Design review of the part built by this model. Coordinates are the model's own, in mm. Coordinates: 2 decimals unless noted, no trailing zeros. Loops run counter-clockwise (first coordinate to the right, second up) from the corner with the lowest first, then second, coordinate; pieces in that order, holes last. Notation, with made-up numbers: (1, 21.25) -> (20, 21.25) arc R10 cw to (20, 26.25) -> close; hole circle Ø6 at (5, 84). An arc over 180 degrees is marked (long way). Use a Markdown table: item, result. Add a question column.
Q1. For probe 1 along Y at (x, z) = (-50, 3.75); probe 2 along X at (y, z) = (38.5, 0.6); probe 3 along Y at (x, z) = (31, 1.25), list the stretches that pass through material, from the lowest coordinate up.
Q2. Take a section at B-B on y = -53. Write out the cut boundary in (x, z), plus the area to 3 significant figures.
Q3. Take a section at A-A on x = 7.5. Write out the cut boundary in (y, z).
Q4. Take a section at D-D on y = -20. Write out the cut boundary in (x, z).
Q5. Take a section at C-C on z = 4.55. Count the separate pieces of the cut face and the enclosed holes in it, plus the area to 3 significant figures.
Q6. Clearance check with a flat-ended pin moving along its axis: pin 1 Ø4.5 at (x, y) = (30, 40) entering from +Z. State where the tip first meets the part, or that it passes through.
Q7. Draft analysis for pull direction X (two halves, no side actions). For faces 1 (the face through (-1, 1, 0)), 2 (the face through (-29.2, 38.5, 3)), 3 (the face through (-62.5, -1, 3)), 4 (the face through (-28.43, 19.35, 2.96)), state which applies: pulls with the +X half, pulls with the -X half, needs draft (parallel to the pull), parting line crosses it, or undercut.
from build123d import *

# Parameters (mm, degrees)
SKETCH1_W           = 125
SKETCH1_H           = 125
SKETCH1_R           = 1.7
SKETCH1_R_2         = 2.65
BOSS_EXTRUDE1_DEPTH = 6
FILLET1_R           = 2.5


with BuildPart() as part:
    # Sketch1 → Boss-Extrude1 (new body)
    with BuildSketch(Plane.XY):
        Rectangle(SKETCH1_W, SKETCH1_H)
        with Locations((-50, 40)):
            Circle(SKETCH1_R, mode=Mode.SUBTRACT)
        with Locations((-30, 40)):
            Circle(SKETCH1_R, mode=Mode.SUBTRACT)
        with Locations((-30, 20)):
            Circle(SKETCH1_R, mode=Mode.SUBTRACT)
        with Locations((-50, 20)):
            Circle(SKETCH1_R, mode=Mode.SUBTRACT)
        with Locations(Location((50, 40, 0), (0, 0, 180))):
            Circle(SKETCH1_R, mode=Mode.SUBTRACT)
        with Locations(Location((50, 20, 0), (0, 0, 180))):
            Circle(SKETCH1_R, mode=Mode.SUBTRACT)
        with Locations(Location((30, 20, 0), (0, 0, 180))):
            Circle(SKETCH1_R, mode=Mode.SUBTRACT)
        with Locations(Location((30, 40, 0), (0, 0, 180))):
            Circle(SKETCH1_R, mode=Mode.SUBTRACT)
        with Locations(Location((-50, -20, 0), (0, 0, 180))):
            Circle(SKETCH1_R, mode=Mode.SUBTRACT)
        with Locations(Location((-30, -20, 0), (0, 0, 180))):
            Circle(SKETCH1_R, mode=Mode.SUBTRACT)
        with Locations(Location((-30, -40, 0), (0, 0, 180))):
            Circle(SKETCH1_R, mode=Mode.SUBTRACT)
        with Locations(Location((-50, -40, 0), (0, 0, 180))):
            Circle(SKETCH1_R, mode=Mode.SUBTRACT)
        with Locations((30, -40)):
            Circle(SKETCH1_R, mode=Mode.SUBTRACT)
        with Locations((30, -20)):
            Circle(SKETCH1_R, mode=Mode.SUBTRACT)
        with Locations((50, -20)):
            Circle(SKETCH1_R, mode=Mode.SUBTRACT)
        with Locations((50, -40)):
            Circle(SKETCH1_R, mode=Mode.SUBTRACT)
        with Locations((7.5, 10)):
            Circle(SKETCH1_R_2, mode=Mode.SUBTRACT)
        with Locations((7.5, -10)):
            Circle(SKETCH1_R_2, mode=Mode.SUBTRACT)
        with Locations((-53, -53)):
            Circle(SKETCH1_R_2, mode=Mode.SUBTRACT)
        with Locations((53, -53)):
            Circle(SKETCH1_R_2, mode=Mode.SUBTRACT)
        with Locations((53, 53)):
            Circle(SKETCH1_R_2, mode=Mode.SUBTRACT)
        with Locations((-53, 53)):
            Circle(SKETCH1_R_2, mode=Mode.SUBTRACT)
    extrude(amount=BOSS_EXTRUDE1_DEPTH)

    # Fillet1
    fillet1_edges = [part.edges().sort_by_distance(p)[0] for p in [
        (-62.5, 62.5, 3),
        (62.5, 62.5, 3),
        (62.5, -62.5, 3),
        (-62.5, -62.5, 3),
    ]]
    fillet(fillet1_edges, radius=FILLET1_R)


solid = part.part
Answer list:
| question | item | result |
|---|---|---|
| 1 | probe 1 | -62.5 to -41.7, -38.3 to -21.7, -18.3 to 18.3, 21.7 to 38.3, 41.7 to 62.5 |
| 1 | probe 2 | -62.5 to -50.8, -49.2 to -30.8, -29.2 to 29.2, 30.8 to 49.2, 50.8 to 62.5 |
| 1 | probe 3 | -62.5 to -41.37, -38.63 to -21.37, -18.63 to 18.63, 21.37 to 38.63, 41.37 to 62.5 |
| 2 | outline | (-62.5, 0) -> (-55.65, 0) -> (-55.65, 6) -> (-62.5, 6) -> close; (-50.35, 0) -> (50.35, 0) -> (50.35, 6) -> (-50.35, 6) -> close; (55.65, 0) -> (62.5, 0) -> (62.5, 6) -> (55.65, 6) -> close |
| 2 | area | 686 mm² |
| 3 | outline | (-62.5, 0) -> (-12.65, 0) -> (-12.65, 6) -> (-62.5, 6) -> close; (-7.35, 0) -> (7.35, 0) -> (7.35, 6) -> (-7.35, 6) -> close; (12.65, 0) -> (62.5, 0) -> (62.5, 6) -> (12.65, 6) -> close |
| 4 | outline | (-62.5, 0) -> (-51.7, 0) -> (-51.7, 6) -> (-62.5, 6) -> close; (-48.3, 0) -> (-31.7, 0) -> (-31.7, 6) -> (-48.3, 6) -> close; (-28.3, 0) -> (28.3, 0) -> (28.3, 6) -> (-28.3, 6) -> close; (31.7, 0) -> (48.3, 0) -> (48.3, 6) -> (31.7, 6) -> close; (51.7, 0) -> (62.5, 0) -> (62.5, 6) -> (51.7, 6) -> close |
| 5 | separate pieces | 1 |
| 5 | enclosed holes | 22 |
| 5 | area | 15,300 mm² |
| 6 | pin 1 | z = 6 |
| 7 | face 1 | needs draft |
| 7 | face 2 | undercut |
| 7 | face 3 | pulls with the -X half |
| 7 | face 4 | undercut |
